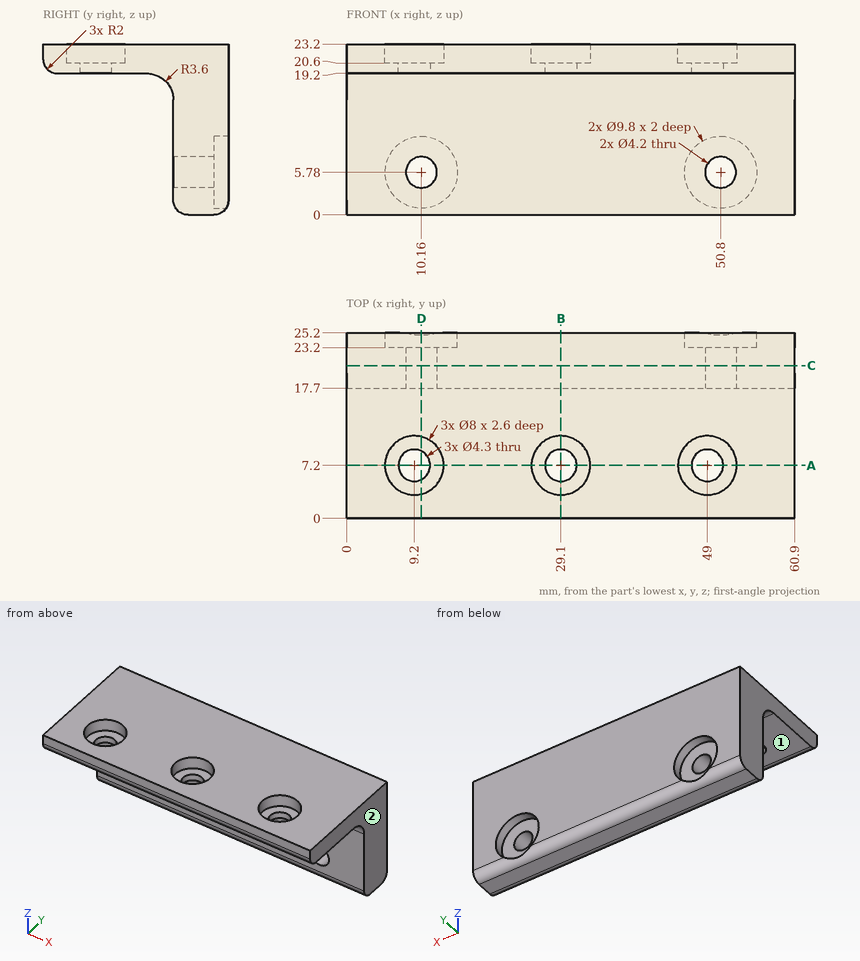
Here's the drawing with two shaded views (mm, measured from the low corner). I have some questions. A direction names the side the tool comes from. Give positions to 0.01 mm unless a question says otherwise; leave off trailing zeros. Order: outer loops, then holes, each group sorted by start corner. A loop starts at its lowest first (then second) coordinate and runs counter-clockwise, first axis right, second up. Notation, with made-up numbers: (23.5, 74) - (48.5, 74) arc R21 ccw to (48.5, 109) - close; hole circle Ø5 at (35.25, -20.5). An arc over 180 degrees is marked (long way). Use a Markdown table: item, result. Add a question column.
Q1. On a 3-axis mill with a long thin cutter (end or side, diameter ignored), from which of +Z, -Z, +X, -X, +Y, -Y can I reach the whole of each face in a straight line? I mean the marked faces 1 and 2. Say none if no direction works.
Q2. If we section it at A-A on y = 7.2: Write out the boundary of the cut face in (x, z).
Q3. If we section it at B-B on x = 29.1: Write out the boundary of the cut face in (y, z).
Q4. If we section it at D-D on x = 10.16: Write out the boundary of the cut face in (y, z).
Q5. If we section it at C-C on y = 20.75: Write out the boundary of the cut face in (x, z).
Q6. Please list where these lines run through material, in increasing order: line 1 along X through (y, z) = (24.4, 5.78); line 2 along Z through (x, y) = (10.16, 20.8); line 3 along Y through (x, z) = (29.1, 21.95).
Q7. I'm going to push flat-ended pins straight in: pin 1 (5 mm diameter, centred on y = 15, z = 12, fed in from +X); pin 2 (7 mm diameter, centred on x = 49, y = 7.2, fed in from -Z); pin 3 (6 mm diameter, centred on x = 10.16, z = 5.78, fed in from -Y); pin 4 (2.5 mm diameter, centred on x = 31, y = 8, fed in from +Z). Where does each tip first touch, or does it pass through?
Answers follow:
| question | item | result |
|---|---|---|
| 1 | face 1 | -Z, +X, -X, -Y |
| 1 | face 2 | +Z, -Z, +X, +Y, -Y |
| 2 | outline | (0, 19.2) - (7.05, 19.2) - (7.05, 20.6) - (5.2, 20.6) - (5.2, 23.2) - (0, 23.2) - close; (11.35, 19.2) - (26.95, 19.2) - (26.95, 20.6) - (25.1, 20.6) - (25.1, 23.2) - (13.2, 23.2) - (13.2, 20.6) - (11.35, 20.6) - close; (31.25, 19.2) - (46.85, 19.2) - (46.85, 20.6) - (45, 20.6) - (45, 23.2) - (33.1, 23.2) - (33.1, 20.6) - (31.25, 20.6) - close; (51.15, 19.2) - (60.9, 19.2) - (60.9, 23.2) - (53, 23.2) - (53, 20.6) - (51.15, 20.6) - close |
| 3 | outline | (0, 21.2) arc R2 ccw to (2, 19.2) - (5.05, 19.2) - (5.05, 20.6) - (3.2, 20.6) - (3.2, 23.2) - (0, 23.2) - close; (9.35, 19.2) - (14.1, 19.2) arc R3.6 cw to (17.7, 15.6) - (17.7, 2) arc R2 ccw to (19.7, 0) - (23.2, 0) arc R2 ccw to (25.2, 2) - (25.2, 23.2) - (11.2, 23.2) - (11.2, 20.6) - (9.35, 20.6) - close |
| 4 | outline | (0, 21.2) arc R2 ccw to (2, 19.2) - (5.28, 19.2) - (5.28, 20.6) - (3.32, 20.6) - (3.32, 23.2) - (0, 23.2) - close; (9.12, 19.2) - (14.1, 19.2) arc R3.6 cw to (17.7, 15.6) - (17.7, 7.88) - (23.2, 7.88) - (23.2, 10.68) - (25.2, 10.68) - (25.2, 23.2) - (11.08, 23.2) - (11.08, 20.6) - (9.12, 20.6) - close; (17.7, 2) arc R2 ccw to (19.7, 0) - (23.2, 0) arc R2 ccw to (24.86, 0.88) - (23.2, 0.88) - (23.2, 3.68) - (17.7, 3.68) - close |
| 5 | outline | (0, 0) - (60.9, 0) - (60.9, 23.2) - (0, 23.2) - close; hole circle Ø4.2 at (10.16, 5.78); hole circle Ø4.2 at (50.8, 5.78) |
| 6 | line 1 | x = 0 to 5.26, 15.06 to 45.9, 55.7 to 60.9 |
| 6 | line 2 | z = 0 to 3.68, 7.88 to 23.2 |
| 6 | line 3 | y = 0 to 3.2, 11.2 to 25.2 |
| 7 | pin 1 | passes through |
| 7 | pin 2 | stops at z = 19.2 |
| 7 | pin 3 | stops at y = 17.7 |
| 7 | pin 4 | stops at z = 20.6 |
